Geometry check sheet. Reference: the model listing, model coordinates, mm. A direction names the side the tool comes from. Round coordinates to 2 decimals unless told otherwise and drop trailing zeros. Order: outer loops, then holes, each group sorted by start corner. A loop starts at its lowest first (then second) coordinate and runs counter-clockwise, first axis right, second up.
(1) Gauge pin test, flat ends, axial feed: P1, Ø2, axis at x = 14, y = -5.5, coming from the -Z side; P2, Ø1.5, axis at y = -2.5, z = -17.5, coming from the -X side; P3, Ø3, axis at x = -13, y = -5, coming from the -Z side. Record the tip position at first contact, or that the pin passes through.
(2) Cross-section at D-D on x = 15. Enter the section's corners in (y, z) (3 decimals).
(3) Cross-section at A-A on x = 0. Enter the section's corners in (y, z), and give its area (3 significant figures).
(4) Cross-section at B-B on y = -5.25. Count the separate pieces of the cut face and the enclosed holes in it, and give its area (3 significant figures).
(5) Draft check along Z on faces 4 (the face through (5.82, -3.13, -10.56)), 5 (the face through (0, -6.35, 20)). Enter one of: pulls with the +Z half, pulls with the -Z half, needs draft (parallel to the pull), parting line crosses it, or undercut.
(6) Thickness scan on L1, parallel to Z at x = 0, y = -2.75; L2, parallel to Z at x = -9.5, y = -2; L3, parallel to X at y = -2.25, z = -7. Record the ranges inside material, lowest first.
(7) Cross-section at C-C on z = -12. Enter the section's corners in (x, y).
(8) Set-up check for faces 1 (the face through (2.394, -3.131, 3.987)), 2 (the face through (-13.66, -4.74, 17.59)), 3 (the face through (5, 0, -5)): record each of +Z, -Z, +X, -X, +Y, -Y from which the full face is reachable in a straight line by a thin tool's end or side.
from build123d import *

# Parameters (mm, degrees)
F1_DEPTH = 6.35
F0_R     = 1.651
F2_DEPTH = 3.175


with BuildPart() as f1:
    # F0 (on Front) → F1 (new body)
    with BuildSketch(Plane.XZ):
        with BuildLine():
            ThreePointArc((11.0264984463, -15.5344401899), (12.6259487856, -14.2649191117), (14.0803208699, -12.831487217))
            Line((14.0803208699, -12.831487217), (3.9810826848, -3.1792186712))
            Line((3.9810826848, -3.1792186712), (0.762, 11.3559151068))
            Line((0.762, 11.3559151068), (0.762, -5.7242254315))
            Line((0.762, -5.7242254315), (11.0264984463, -15.5344401899))
        make_face()
        with BuildLine():
            Line((-3.9805361158, -3.1797711993), (-14.0807017487, -12.8310692565))
            ThreePointArc((-14.0807017487, -12.8310692565), (-12.6263635982, -14.2645519483), (-11.0269407935, -15.5341261981))
            Line((-11.0269407935, -15.5341261981), (-0.762, -5.725375853))
            Line((-0.762, -5.725375853), (-0.762, 11.3895507529))
            Line((-0.762, 11.3895507529), (-3.9805361158, -3.1797711993))
        make_face()
        with BuildLine():
            ThreePointArc((-17.8734776092, 18.047127144), (-9.7768519659, -23.4429768937), (25.4, 0))
            ThreePointArc((25.4, 0), (23.4429768937, 9.7768519659), (17.8734776092, 18.047127144))
            Line((17.8734776092, 18.047127144), (13.9408592709, 12.9828711304))
            ThreePointArc((13.9408592709, 12.9828711304), (17.7267575872, 6.9759992434), (19.05, 0))
            ThreePointArc((19.05, 0), (17.7641860575, -6.8801303559), (14.0803208699, -12.831487217))
            ThreePointArc((14.0803208699, -12.831487217), (12.6259487856, -14.2649191117), (11.0264984463, -15.5344401899))
            ThreePointArc((11.0264984463, -15.5344401899), (-0.0002712295, -19.0499999981), (-11.0269407935, -15.5341261981))
            ThreePointArc((-11.0269407935, -15.5341261981), (-12.6263635982, -14.2645519483), (-14.0807017487, -12.8310692565))
            ThreePointArc((-14.0807017487, -12.8310692565), (-19.0497204722, 0.1031985072), (-13.9408592709, 12.9828711304))
            Line((-13.9408592709, 12.9828711304), (-17.8734776092, 18.047127144))
        make_face()
    extrude(amount=F1_DEPTH)



with BuildPart() as f1b:
    # F0 (on Front) → F1, piece 2 (new body)
    with BuildSketch(Plane.XZ):
        with BuildLine():
            Line((11.684, 15.0461504711), (15.5786666667, 20.0615339615))
            ThreePointArc((15.5786666667, 20.0615339615), (0, 25.4), (-15.5786666667, 20.0615339615))
            Line((-15.5786666667, 20.0615339615), (-11.684, 15.0461504711))
            ThreePointArc((-11.684, 15.0461504711), (0, 19.05), (11.684, 15.0461504711))
        make_face()
        with Locations((0, 22.225)):
            Circle(F0_R, mode=Mode.SUBTRACT)
    extrude(amount=F1_DEPTH)


with BuildPart() as f1_1:
    add(f1.part)

    add(f1b.part)  # F2 merges F1b
    # F0 (on Front) → F2 (join)
    with BuildSketch(Plane.XZ):
        with BuildLine():
            ThreePointArc((-15.5786666667, 20.0615339615), (-16.7563703668, 19.0888462755), (-17.8734776092, 18.047127144))
            Line((-17.8734776092, 18.047127144), (-13.9408592709, 12.9828711304))
            ThreePointArc((-13.9408592709, 12.9828711304), (-12.8538956575, 14.0598672265), (-11.684, 15.0461504711))
            Line((-11.684, 15.0461504711), (-15.5786666667, 20.0615339615))
        make_face()
        with BuildLine():
            Line((13.9408592709, 12.9828711304), (17.8734776092, 18.047127144))
            ThreePointArc((17.8734776092, 18.047127144), (16.7563703668, 19.0888462755), (15.5786666667, 20.0615339615))
            Line((15.5786666667, 20.0615339615), (11.684, 15.0461504711))
            ThreePointArc((11.684, 15.0461504711), (12.8538956575, 14.0598672265), (13.9408592709, 12.9828711304))
        make_face()
    extrude(amount=F2_DEPTH)


solid = f1_1.part
Found:
1. P1: stops at z = -21.82
1. P2: stops at x = -19.09
1. P3: stops at z = -22.65
2. outline: (-6.35, -20.498) - (0, -20.498) - (0, -11.743) - (-6.35, -11.743) - close; (-6.35, 11.743) - (0, 11.743) - (0, 20.498) - (-6.35, 20.498) - (-6.35, 19.316) - (-3.175, 19.316) - (-3.175, 14.347) - (-6.35, 14.347) - close
3. outline: (-6.35, -25.4) - (0, -25.4) - (0, -19.05) - (-6.35, -19.05) - close; (-6.35, 19.05) - (0, 19.05) - (0, 20.57) - (-6.35, 20.57) - close; (-6.35, 23.88) - (0, 23.88) - (0, 25.4) - (-6.35, 25.4) - close
3. area: 59.7 mm2
4. separate pieces: 2
4. enclosed holes: 1
4. area: 1,010 mm2
5. face 4: undercut
5. face 5: needs draft
6. L1: z = -25.4 to -19.05, 19.05 to 20.57, 23.88 to 25.4
6. L2: z = -23.56 to -16.51, -14.08 to -8.45, 16.51 to 23.56
6. L3: x = -24.42 to -17.72, -7.98 to -2.1, 2.1 to 7.98, 17.72 to 24.42
7. outline: (-22.39, -6.35) - (-14.8, -6.35) - (-14.8, 0) - (-22.39, 0) - close; (-13.21, -6.35) - (-7.33, -6.35) - (-7.33, 0) - (-13.21, 0) - close; (7.33, -6.35) - (13.21, -6.35) - (13.21, 0) - (7.33, 0) - close; (14.8, -6.35) - (22.39, -6.35) - (22.39, 0) - (14.8, 0) - close
8. face 1: +Y, -Y
8. face 2: -Y
8. face 3: +Z, -Z, +X, -X, +Y
